```python
from build123d import *

# Parameters (mm, degrees)
SKETCH1_R                  = 54.76875
BOSS_EXTRUDE1_DEPTH        = 37.30625
SKETCH2_R                  = 51.59375
CUT_EXTRUDE1_DEPTH         = 30.95625
SKETCH3_R                  = 1.5875
CUT_EXTRUDE2_DEPTH         = 3.175
SKETCH4_R                  = 17.4625
CUT_EXTRUDE3_DEPTH         = 84.411757967
BOSS_EXTRUDE2_START        = -35.71875
BOSS_EXTRUDE2_DEPTH        = 35.71875
F_1_0_228_DIAMETER_HOLE1_D = 5.7912


with BuildPart() as part:
    # Sketch1 → Boss-Extrude1 (new body)
    with BuildSketch(Plane.XY):
        Circle(SKETCH1_R)
    extrude(amount=BOSS_EXTRUDE1_DEPTH)

    # Sketch2 → Cut-Extrude1 (cut)
    with BuildSketch(Plane.XY.offset(37.30625)):
        Circle(SKETCH2_R)
    extrude(amount=-CUT_EXTRUDE1_DEPTH, mode=Mode.SUBTRACT)

    # Sketch3 → Cut-Extrude2 (cut)
    with BuildSketch(Plane.XY.offset(6.35)):
        with Locations((-47.625, 0)):
            Circle(SKETCH3_R)
        with Locations((-46.584279485, 9.901794275)):
            Circle(SKETCH3_R)
        with Locations((-43.50760242, 19.370832626)):
            Circle(SKETCH3_R)
        with Locations((-38.529434357, 27.99327264)):
            Circle(SKETCH3_R)
        with Locations((-31.867345128, 35.392272313)):
            Circle(SKETCH3_R)
        with Locations((-23.8125, 41.244459855)):
            Circle(SKETCH3_R)
        with Locations((-14.716934357, 45.294066589)):
            Circle(SKETCH3_R)
        with Locations((-4.978168063, 47.364105267)):
            Circle(SKETCH3_R)
        with Locations((4.978168063, 47.364105267)):
            Circle(SKETCH3_R)
        with Locations((14.716934357, 45.294066589)):
            Circle(SKETCH3_R)
        with Locations((23.8125, 41.244459855)):
            Circle(SKETCH3_R)
        with Locations((31.867345128, 35.392272313)):
            Circle(SKETCH3_R)
        with Locations((38.529434357, 27.99327264)):
            Circle(SKETCH3_R)
        with Locations((43.50760242, 19.370832626)):
            Circle(SKETCH3_R)
        with Locations((46.584279485, 9.901794275)):
            Circle(SKETCH3_R)
        with Locations((47.625, 0)):
            Circle(SKETCH3_R)
        with Locations((46.584279485, -9.901794275)):
            Circle(SKETCH3_R)
        with Locations((43.50760242, -19.370832626)):
            Circle(SKETCH3_R)
        with Locations((38.529434357, -27.99327264)):
            Circle(SKETCH3_R)
        with Locations((31.867345128, -35.392272313)):
            Circle(SKETCH3_R)
        with Locations((23.8125, -41.244459855)):
            Circle(SKETCH3_R)
        with Locations((14.716934357, -45.294066589)):
            Circle(SKETCH3_R)
        with Locations((4.978168063, -47.364105267)):
            Circle(SKETCH3_R)
        with Locations((-4.978168063, -47.364105267)):
            Circle(SKETCH3_R)
        with Locations((-14.716934357, -45.294066589)):
            Circle(SKETCH3_R)
        with Locations((-23.8125, -41.244459855)):
            Circle(SKETCH3_R)
        with Locations((-31.867345128, -35.392272313)):
            Circle(SKETCH3_R)
        with Locations((-38.529434357, -27.99327264)):
            Circle(SKETCH3_R)
        with Locations((-43.50760242, -19.370832626)):
            Circle(SKETCH3_R)
        with Locations((-46.584279485, -9.901794275)):
            Circle(SKETCH3_R)
    extrude(amount=-CUT_EXTRUDE2_DEPTH, mode=Mode.SUBTRACT)

    # Sketch4 → Cut-Extrude3 (cut, through all)
    with BuildSketch(Plane.XY.offset(6.35)):
        Circle(SKETCH4_R)
    extrude(amount=-CUT_EXTRUDE3_DEPTH, mode=Mode.SUBTRACT)

    # Sketch7 → Boss-Extrude2 (add)
    with BuildSketch(Plane.XY.offset(37.30625).offset(BOSS_EXTRUDE2_START)):
        with BuildLine():
            Line((-54.561291868, 4.7625), (-59.53125, 4.7625))
            ThreePointArc((-59.53125, 4.7625), (-64.29375, 0), (-59.53125, -4.7625))
            Line((-59.53125, -4.7625), (-54.561291868, -4.7625))
            ThreePointArc((-54.561291868, -4.7625), (-54.76875, 0), (-54.561291868, 4.7625))
        make_face()
        with BuildLine():
            Line((-4.7625, 59.53125), (-4.7625, 54.561291868))
            ThreePointArc((-4.7625, 54.561291868), (0, 54.76875), (4.7625, 54.561291868))
            Line((4.7625, 54.561291868), (4.7625, 59.53125))
            ThreePointArc((4.7625, 59.53125), (0, 64.29375), (-4.7625, 59.53125))
        make_face()
        with BuildLine():
            ThreePointArc((4.7625, -54.561291868), (0, -54.76875), (-4.7625, -54.561291868))
            Line((-4.7625, -54.561291868), (-4.7625, -59.53125))
            ThreePointArc((-4.7625, -59.53125), (0, -64.29375), (4.7625, -59.53125))
            Line((4.7625, -59.53125), (4.7625, -54.561291868))
        make_face()
        with BuildLine():
            Line((59.53125, 4.7625), (54.561291868, 4.7625))
            ThreePointArc((54.561291868, 4.7625), (54.76875, 0), (54.561291868, -4.7625))
            Line((54.561291868, -4.7625), (59.53125, -4.7625))
            ThreePointArc((59.53125, -4.7625), (64.29375, 0), (59.53125, 4.7625))
        make_face()
    extrude(amount=BOSS_EXTRUDE2_DEPTH)

    # #1 (0.228) Diameter Hole1 (through all)
    with Locations(Plane.XY.offset(37.30625)):
        with Locations((-59.53125, 0), (0, 59.53125), (59.53125, 0), (0, -59.53125)):
            Hole(F_1_0_228_DIAMETER_HOLE1_D / 2)


solid = part.part
```
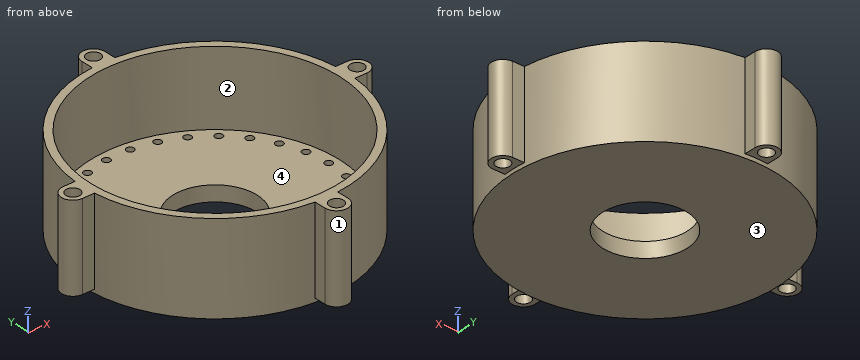
The listing builds one solid part. Answer for the finished solid, in the listing's coordinates (mm). Face numbers are marked on the shaded views. Give positions to 0.01 mm unless a question says otherwise; leave off trailing zeros. Order: outer loops, then holes, each group sorted by start corner. A loop starts at its lowest first (then second) coordinate and runs counter-clockwise, first axis right, second up.
1) Find section C-C on z = 12. Write down the section's boundary in (x, y) (1 decimal), then the cut area to 3 significant figures.
Reported:
outline: (-59.5, -4.8) - (-54.6, -4.8) arc R54.8 ccw to (-4.8, -54.6) - (-4.8, -59.5) arc R4.8 ccw to (4.8, -59.5) - (4.8, -54.6) arc R54.8 ccw to (54.6, -4.8) - (59.5, -4.8) arc R4.8 ccw to (59.5, 4.8) - (54.6, 4.8) arc R54.8 ccw to (4.8, 54.6) - (4.8, 59.5) arc R4.8 ccw to (-4.8, 59.5) - (-4.8, 54.6) arc R54.8 ccw to (-54.6, 4.8) - (-59.5, 4.8) arc R4.8 ccw to start; hole circle Ø5.8 at (-59.5, 0); hole circle Ø103.2 at (0, 0); hole circle Ø5.8 at (0, -59.5); hole circle Ø5.8 at (0, 59.5); hole circle Ø5.8 at (59.5, 0)
area: 1,280 mm2
2) Determine the mould class of the marked faces 1, 2, 3 and 4 for opening direction Y: pulls with the +Y half, pulls with the -Y half, needs draft (parallel to the pull), parting line crosses it, or undercut.
Reported:
face 1: pulls with the -Y half
face 2: undercut
face 3: needs draft
face 4: undercut
3) Find section B-B on y = 0. Give the number of separate pieces and of enclosed holes in the cut face, then the cut area to 3 significant figures.
Reported:
separate pieces: 4
enclosed holes: 0
area: 917 mm2
4) Find section A-A on x = 0. Write down the section's boundary in (y, z), then the cut area to 3 significant figures.
Reported:
outline: (-64.29, 1.59) - (-62.43, 1.59) - (-62.43, 37.31) - (-64.29, 37.31) - close; (-56.64, 1.59) - (-54.77, 1.59) - (-54.77, 0) - (-17.46, 0) - (-17.46, 6.35) - (-51.59, 6.35) - (-51.59, 37.31) - (-56.64, 37.31) - close; (17.46, 0) - (54.77, 0) - (54.77, 1.59) - (56.64, 1.59) - (56.64, 37.31) - (51.59, 37.31) - (51.59, 6.35) - (17.46, 6.35) - close; (62.43, 1.59) - (64.29, 1.59) - (64.29, 37.31) - (62.43, 37.31) - close
area: 937 mm2
5) Consider line 1 along Y through (x, z) = (0, 3); line 2 along Y through (x, z) = (0, 22); line 3 along Z through (x, y) = (-6.5, -44). Determine where each line is inside the solid, lowest interval first.
Reported:
line 1: y = -64.29 to -62.43, -56.64 to -17.46, 17.46 to 56.64, 62.43 to 64.29
line 2: y = -64.29 to -62.43, -56.64 to -51.59, 51.59 to 56.64, 62.43 to 64.29
line 3: z = 0 to 6.35
6) Given P1, Ø12, axis at y = 43, z = 22, coming from the +X side; P2, Ø4, axis at x = 58, z = 12, coming from the +Y side; P3, Ø2.5, axis at x = -31.5, y = 35.5, coming from the +Z side; P4, Ø4, axis at x = 37.5, y = 1.5, coming from the -Z side, each flat-ended and moving along its own axis, determine where each tip first touches the part or whether it passes through.
Reported:
P1: stops at x = 40.38
P2: stops at y = 4.76
P3: stops at z = 6.35
P4: stops at z = 0
7) Find section D-D on x = -20. Write down the section's boundary in (y, z), then the cut area to 3 significant figures.
Reported:
outline: (-50.99, 0) - (50.99, 0) - (50.99, 37.31) - (47.56, 37.31) - (47.56, 6.35) - (-47.56, 6.35) - (-47.56, 37.31) - (-50.99, 37.31) - close
area: 860 mm2
